The listing builds one solid part. Answer for the finished solid, in the listing's coordinates (mm). Face numbers are marked on the shaded views. Coordinates: 2 decimals unless noted, no trailing zeros. Order: outer loops, then holes, each group sorted by start corner. A loop starts at its lowest first (then second) coordinate and runs counter-clockwise, first axis right, second up. Notation, with made-up numbers: (86.25, 39) - (116.25, 39) arc R33 cw to (116.25, 75) - close; hole circle Ø9 at (-13, 83). An arc over 180 degrees is marked (long way). Use one line per item in the form item = value. Start each with the question number.
Item 1: Section A-A, the plane x = 81.5 is taken. Write down the section's boundary in (y, z), and give its area (3 significant figures).
Item 2: Consider line 1 along X through (y, z) = (19, 7.5); line 2 along Y through (x, z) = (72, -7); line 3 along Y through (x, z) = (110, -10). Determine where each line is inside the solid, lowest interval first. Write a range as [from, to].
Item 3: Each of these flat-tipped pins is pushed along its axis until it touches: pin 1 Ø5 at (x, z) = (-13.5, -2) entering from +Y; pin 2 Ø12 at (y, z) = (9, 16) entering from -X; pin 3 Ø8 at (y, z) = (13, 25) entering from -X. Where does it stop, or does it pass through?
Item 4: The mould has two halves that part along X. Classify the marked faces 1, 2 and 3: released by +X, released by -X, zero draft, split by the parting line, or undercut.
from build123d import *

# Parameters (mm, degrees)
BOSS_EXTRUDE1_DEPTH = 20
CUT_EXTRUDE1_DEPTH  = 7.5
FILLET1_R           = 40
FILLET2_R           = 1
FILLET3_R           = 2
SKETCH6_R           = 1
CUT_EXTRUDE2_DEPTH  = 15


with BuildPart() as part:
    # Sketch1 → Boss-Extrude1 (new body)
    with BuildSketch(Plane(origin=(0, 0, 0), x_dir=(1, 0, 0), z_dir=(0, 1, 0))):
        with BuildLine():
            Line((-100, 37.5), (100, 37.5))
            ThreePointArc((100, 37.5), (137.5, 0), (100, -37.5))
            Line((100, -37.5), (-100, -37.5))
            ThreePointArc((-100, -37.5), (-137.5, 0), (-100, 37.5))
        make_face()
    extrude(amount=BOSS_EXTRUDE1_DEPTH)

    # Sketch2 → Cut-Extrude1 (cut)
    with BuildSketch(Plane(origin=(0, 20, 0), x_dir=(1, 0, 0), z_dir=(0, 1, 0))):
        with BuildLine():
            Line((-100, -35.5), (100, -35.5))
            ThreePointArc((100, -35.5), (135.5, 0), (100, 35.5))
            Line((100, 35.5), (-100, 35.5))
            ThreePointArc((-100, 35.5), (-135.5, 0), (-100, -35.5))
        make_face()
    extrude(amount=-CUT_EXTRUDE1_DEPTH, mode=Mode.SUBTRACT)

    # Fillet1
    # the kernel refuses this fillet: 40 mm, written as the material it adds along each edge
    with BuildSketch(Plane(origin=(100, 12.5, -35.5), x_dir=(0, 1, 0), z_dir=(-1, 0, 0)), Plane(origin=(-100, 12.5, 35.5), x_dir=(0, 1, 0), z_dir=(1, 0, 0))) as fillet1_piece_1:
        with BuildLine():
            CenterArc((40, -23.318447633), FILLET1_R, 144.340912304, 35.659087696)
            Line((0, -23.318447633), (-0.8, -23.318447633))
            Line((-0.8, -23.318447633), (-0.8, 0))
            Line((-0.8, 0), (0, 0.8))
            ThreePointArc((0, 0.8), (3.75, 0.8), (6.85, 0.466368953))
            Line((6.85, 0.466368953), (7.5, 0))
        make_face()
    extrude(amount=200)
    with BuildSketch(Plane(origin=(-100, 12.5, 0), x_dir=(0, 0, -1), z_dir=(1, 0, 0))) as fillet1_piece_2:
        with BuildLine():
            CenterArc((12.181552367, 40), FILLET1_R, 270, 35.659087696)
            Line((12.181552367, 0), (12.181552367, -0.8))
            Line((12.181552367, -0.8), (35.5, -0.8))
            Line((35.5, -0.8), (36.3, 0))
            ThreePointArc((36.3, 0), (36.3, 3.75), (35.966368953, 6.85))
            Line((35.966368953, 6.85), (35.5, 7.5))
        make_face()
    revolve(axis=Axis((-100, 12.5, 0), (0, 1, 0)), revolution_arc=180)
    with BuildSketch(Plane(origin=(100, 12.5, 0), x_dir=(0, 0, 1), z_dir=(-1, 0, 0))) as fillet1_piece_3:
        with BuildLine():
            CenterArc((12.181552367, 40), FILLET1_R, 270, 35.659087696)
            Line((12.181552367, 0), (12.181552367, -0.8))
            Line((12.181552367, -0.8), (35.5, -0.8))
            Line((35.5, -0.8), (36.3, 0))
            ThreePointArc((36.3, 0), (36.3, 3.75), (35.966368953, 6.85))
            Line((35.966368953, 6.85), (35.5, 7.5))
        make_face()
    revolve(axis=Axis((100, 12.5, 0), (0, 1, 0)), revolution_arc=180)

    # Fillet2
    fillet2_edges = [part.edges().sort_by_distance(p)[0] for p in [
        (137.5, 20, 0),
        (0, 20, -37.5),
        (-135.5, 20, 0),
        (0, 20, 35.5),
        (135.5, 20, 0),
        (0, 20, -35.5),
        (-137.5, 20, 0),
        (0, 20, 37.5),
    ]]
    fillet(fillet2_edges, radius=FILLET2_R)

    # Fillet3
    fillet3_edges = [part.edges().sort_by_distance(p)[0] for p in [
        (0, 0, -37.5),
        (137.5, 0, 0),
        (0, 0, 37.5),
        (-137.5, 0, 0),
    ]]
    fillet(fillet3_edges, radius=FILLET3_R)

    # Sketch4 → Revolve1 (revolve)
    with BuildSketch(Plane.XY):
        with BuildLine():
            Line((-100, 12), (-100, 42))
            ThreePointArc((-100, 42), (-115, 27), (-100, 12))
        make_face()
    revolve(axis=Axis((-100, 12, 0), (0, 1, 0)))

    # Sketch6 → Cut-Extrude2 (cut)
    with BuildSketch(Plane(origin=(-25.893398282, -25.893398282, 0), x_dir=(0.7071067811865488, -0.7071067811865464, 0), z_dir=(0.7071067811865464, 0.7071067811865488, 0))):
        with Locations(Location((-89.802561211, 0, 0), (0, 0, 180))):
            Circle(SKETCH6_R)
    extrude(amount=-CUT_EXTRUDE2_DEPTH, mode=Mode.SUBTRACT)


solid = part.part
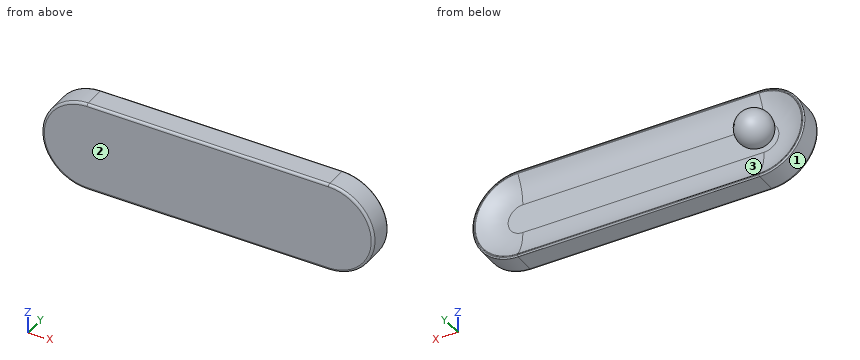
Response:
q1.outline = (0, -35.5) arc R2 ccw to (2, -37.5) - (19, -37.5) arc R1 ccw to (20, -36.5) - (20, -35.82) arc R1 ccw to (19.82, -35.24) arc R40 cw to (12.5, -12.18) - (12.5, 12.18) arc R40 cw to (19.82, 35.24) arc R1 ccw to (20, 35.82) - (20, 36.5) arc R1 ccw to (19, 37.5) - (2, 37.5) arc R2 ccw to (0, 35.5) - close
q1.area = 1,080 mm2
q2.line_1 = [-136.74, -133.2], [-110.23, -89.77], [133.2, 136.74]
q2.line_2 = [0, 12.5]
q2.line_3 = [0, 12.55]
q3.pin_1 = 12.5
q3.pin_2 = -136.14
q3.pin_3 = -131.07
q4.face_1 = released by -X
q4.face_2 = zero draft
q4.face_3 = undercut
